```python
from build123d import *

# Parameters (mm, degrees)
BOSS_EXTRUDE1_DEPTH = 4.445
SKETCH2_W           = 10.16
SKETCH2_H           = 4.953
CUT_EXTRUDE1_DEPTH  = 2.54
FILLET1_R           = 2.54
FILLET2_R           = 7.62


with BuildPart() as part:
    # Sketch1 → Boss-Extrude1 (new body)
    with BuildSketch(Plane.XY):
        Polygon((0, 0), (17.78, 0), (17.78, -14.478), (10.16, -14.478), (10.16, -8.89), (0, -8.89), align=None)
    extrude(amount=BOSS_EXTRUDE1_DEPTH)

    # Sketch2 → Cut-Extrude1 (cut)
    with BuildSketch(Plane.XY.offset(4.445)):
        with Locations((5.08, -4.445)):
            Rectangle(SKETCH2_W, SKETCH2_H)
    extrude(amount=-CUT_EXTRUDE1_DEPTH, mode=Mode.SUBTRACT)

    # Fillet1
    fillet1_edges = [part.edges().sort_by_distance(p)[0] for p in [
        (10.16, -8.89, 2.2225),
    ]]
    fillet(fillet1_edges, radius=FILLET1_R)

    # Fillet2
    fillet2_edges = [part.edges().sort_by_distance(p)[0] for p in [
        (17.78, 0, 2.2225),
    ]]
    fillet(fillet2_edges, radius=FILLET2_R)


solid = part.part
```
Geometry check sheet. Reference: the model listing, model coordinates, mm. A direction names the side the tool comes from. Coordinates: 2 decimals unless noted, no trailing zeros. Order: outer loops, then holes, each group sorted by start corner. A loop starts at its lowest first (then second) coordinate and runs counter-clockwise, first axis right, second up.
Item 1: Section check D-D (z = 3.9). Enter the section's corners in (x, y).
Item 2: Mould release check, pull along Y, two halves, no side actions. Record for faces 1 (the flat face through (5, -1.969, 3)), 2 (the flat face through (10.16, -4, 3)), 3 (the flat face through (5, 0, 2)), 4 (the flat face through (11, -7, 4.445)): released by +Y, released by -Y, zero draft, split by the parting line, or undercut.
Item 3: Scan lines: line 1 along Y through (x, z) = (5.25, 2.75); line 2 along Y through (x, z) = (6.25, 1.45); line 3 along Z through (x, y) = (2, -2.75) (3 decimals). Record each from-to range of solid material in increasing order.
Item 4: Section check C-C (y = -2.5). Enter the section's corners in (x, z) (3 decimals), plus the area to 3 significant figures.
Item 5: Section check B-B (x = 6.5). Enter the section's corners in (y, z) (1 decimal), plus the area to 3 significant figures.
Item 6: Section check A-A (z = 0.3). Enter the section's corners in (x, y).
Item 7: Depth check by flat-ended pin: pin 1 (0.8 mm diameter, centred on x = 5.5, z = 3.5, fed in from -Y); pin 2 (1.5 mm diameter, centred on x = 5.5, y = -5.5, fed in from +Z) (3 decimals); pin 3 (2 mm diameter, centred on y = -4.5, z = 3.5, fed in from -X). Enter the tip coordinate at first touch or a pass-through.
Item 8: Tool access check on faces 5 (the flat face through (0, -4.5, 1.7)), 6 (the flat face through (5, -4, 1.905)), 7 (the flat face through (4, -8.89, 2)). Record the directions out of +Z, -Z, +X, -X, +Y, -Y that give a thin tool (end or side, any length) a straight path to the whole face; none if there is none.
Check sheet entries:
1. outline: (0, -8.89) - (7.62, -8.89) arc R2.54 cw to (10.16, -11.43) - (10.16, -14.48) - (17.78, -14.48) - (17.78, -7.62) arc R7.62 ccw to (10.16, 0) - (0, 0) - (0, -1.97) - (10.16, -1.97) - (10.16, -6.92) - (0, -6.92) - close
2. face 1: undercut
2. face 2: undercut
2. face 3: released by +Y
2. face 4: zero draft
3. line 1: y = -8.89 to -6.92, -1.97 to 0
3. line 2: y = -8.89 to 0
3. line 3: z = 0 to 1.905
4. outline: (0, 0) - (15.804, 0) - (15.804, 4.445) - (10.16, 4.445) - (10.16, 1.905) - (0, 1.905) - close
4. area: 44.4 mm2
5. outline: (-8.9, 0) - (0, 0) - (0, 4.4) - (-2, 4.4) - (-2, 1.9) - (-6.9, 1.9) - (-6.9, 4.4) - (-8.9, 4.4) - close
5. area: 26.9 mm2
6. outline: (0, -8.89) - (7.62, -8.89) arc R2.54 cw to (10.16, -11.43) - (10.16, -14.48) - (17.78, -14.48) - (17.78, -7.62) arc R7.62 ccw to (10.16, 0) - (0, 0) - close
7. pin 1: stops at y = -8.89
7. pin 2: stops at z = 1.905
7. pin 3: stops at x = 10.16
8. face 5: +Z, -Z, -X, +Y, -Y
8. face 6: +Z, -X
8. face 7: +Z, -Z, -X, -Y
